Could you check a few things on this model? Use its own coordinates, in mm. A direction names the side the tool comes from. Round coordinates to 2 decimals unless told otherwise and drop trailing zeros. Loops run counter-clockwise (first coordinate to the right, second up) from the corner with the lowest first, then second, coordinate; pieces in that order, holes last. Notation, with made-up numbers: (-12, 60) -> (11, 60) arc R16 cw to (11, 90) -> close; hole circle Ø8 at (-9, 63). An arc over 180 degrees is marked (long way). Use CSV: the item, a comma, the result in double quotes. Start each with the question number.
```python
from build123d import *

# Parameters (mm, degrees)
F0_W     = 914.4
F0_H     = 914.4
F1_DEPTH = 50.8
F2_W     = 101.6
F2_H     = 101.6
F3_DEPTH = 1219.2
F4_W     = 304.8
F4_H     = 355.6
F5_DEPTH = 228.6
F6_W     = 203.2
F6_H     = 355.6
F7_DEPTH = 177.8
F8_R     = 25.39999


# Not quite as in the source:
# - a fillet or chamfer is up to 0.001 mm smaller than in the source, because OpenCascade refuses the exact size
# - a feature names something its author has since deleted; it is built from what else it names


with BuildPart() as f1:
    # F0 (on Top) → F1 (new body)
    with BuildSketch(Plane.XY):
        with Locations((11.3640455229, 0)):
            Rectangle(F0_W, F0_H)
    extrude(amount=F1_DEPTH)

    # F2 (on face) → F3 (join)
    with BuildSketch(Plane(origin=(0, 0, 0), x_dir=(1, 0, 0), z_dir=(0, 0, -1))):
        Rectangle(F2_W, F2_H)
    extrude(amount=-F3_DEPTH)

    # F4 (on face) → F5 (join)
    with BuildSketch(Plane.XY.offset(1219.2)):
        Rectangle(F4_W, F4_H)
    extrude(amount=F5_DEPTH)

    # F6 (on face) → F7 (cut)
    with BuildSketch(Plane.XY.offset(1447.8)):
        Rectangle(F6_W, F6_H)
    extrude(amount=-F7_DEPTH, mode=Mode.SUBTRACT)

    # F8 (radius 25.4 in the source; OpenCascade refuses exactly that, so slightly less here)
    f8_edges = [f1.edges().sort_by_distance(p)[0] for p in [
        (-152.4, 0, 1447.8),
        (-101.6, 0, 1447.8),
        (101.6, 0, 1447.8),
        (152.4, 0, 1447.8),
    ]]
    fillet(f8_edges, radius=F8_R)


solid = f1.part
```
1. If I drill on L1, parallel to X at y = 27, z = 716.5; L2, parallel to Z at x = -348, y = -198; L3, parallel to Z at x = -41.5, y = 13, over which ranges is the centre line in solid material (lowest first)?
2. Will these pins go through, and if not, where does the flat tip stop? pin 1 (1.5 mm diameter, centred on x = 69, y = -11.5, fed in from -Z); pin 2 (10 mm diameter, centred on x = 2.5, z = 323.5, fed in from -Y); pin 3 (10 mm diameter, centred on x = 169, y = 82, fed in from +Z); pin 4 (10 mm diameter, centred on y = -174.5, z = 1234, fed in from -X).
3. Suppose I cut it at D-D (y = -345). List the corners of the cut face in (x, z) for me.
4. Suppose I cut it at A-A (z = 1343). List the corners of the cut face in (x, y) for me.
5. For faces 5 (the face through (50.8, 1, 627)), 6 (the face through (-1, 50.8, 627)), 7 (the face through (152.4, -2, 1319)), which set-ups out of +Z, -Z, +X, -X, +Y, -Y let a thin tool reach every point of the face, with its end or its side?
6. Suppose I cut it at C-C (x = -234.5). List the corners of the cut face in (y, z) for me, then the cut area to 3 significant figures.
7. We'd pull the mould along Z, two halves only. Please class faces 1 (the face through (-50.8, 1, 627)), 2 (the face through (5, -6, 0)), 3 (the face through (66, 2, 1219.2)), 4 (the face through (5, -457.2, 25)): pulls with the +Z half, pulls with the -Z half, needs draft (parallel to the pull), parting line crosses it, or undercut.
Geometry check:
1,L1,"x = -50.8 to 50.8"
1,L2,"z = 0 to 50.8"
1,L3,"z = 0 to 1270"
2,pin 1,"stops at z = 0"
2,pin 2,"stops at y = -50.8"
2,pin 3,"stops at z = 50.8"
2,pin 4,"stops at x = -152.4"
3,outline,"(-445.84, 0) -> (468.56, 0) -> (468.56, 50.8) -> (-445.84, 50.8) -> close"
4,outline,"(-152.4, -177.8) -> (-101.6, -177.8) -> (-101.6, 177.8) -> (-152.4, 177.8) -> close; (101.6, -177.8) -> (152.4, -177.8) -> (152.4, 177.8) -> (101.6, 177.8) -> close"
5,face 5,"+X, +Y, -Y"
5,face 6,"+X, -X, +Y"
5,face 7,"+Z, +X, +Y, -Y"
6,outline,"(-457.2, 0) -> (457.2, 0) -> (457.2, 50.8) -> (-457.2, 50.8) -> close"
6,area,"46,500 mm²"
7,face 1,"undercut"
7,face 2,"pulls with the -Z half"
7,face 3,"undercut"
7,face 4,"needs draft"
